The listing builds one solid part. Answer for the finished solid, in the listing's coordinates (mm). A direction names the side the tool comes from. Give positions to 0.01 mm unless a question says otherwise; leave off trailing zeros. Write each loop counter-clockwise with the first axis right and the second up, starting at its lowest first coordinate (ties: lowest second). Pieces come first, ordered by that corner, then holes. Notation, with made-up numbers: (62.5, -28.5) -> (83.5, -28.5) arc R24 cw to (83.5, -15.5) -> close; hole circle Ø1 at (-38.75, 55). An arc over 180 degrees is marked (long way). Use CSV: the item, a comma, the result in double quotes. Start each with the question number.
from build123d import *

# Parameters (mm, degrees)
SKETCH1_R           = 5.08
BOSS_EXTRUDE1_DEPTH = 7.62
SKETCH2_W           = 15.638324702
SKETCH2_H           = 10.16
CUT_EXTRUDE1_DEPTH  = 87.890649094
FILLET1_R           = 12.7
FILLET2_R           = 5.08


with BuildPart() as part:
    # Sketch1 → Boss-Extrude1 (new, symmetric)
    with BuildSketch(Plane(origin=(0, 0, 0), x_dir=(1, 0, 0), z_dir=(0, 1, 0))):
        with BuildLine():
            Line((2.735663722, 7.112), (8.018324702, 5.08))
            Line((8.018324702, 5.08), (8.018324702, 3.81))
            Line((8.018324702, 3.81), (68.181675298, 3.81))
            Line((68.181675298, 3.81), (68.181675298, 5.08))
            Line((68.181675298, 5.08), (73.464336278, 7.112))
            ThreePointArc((73.464336278, 7.112), (83.82, 0), (73.464336278, -7.112))
            Line((73.464336278, -7.112), (68.181675298, -5.08))
            Line((68.181675298, -5.08), (68.181675298, -3.81))
            Line((68.181675298, -3.81), (8.018324702, -3.81))
            Line((8.018324702, -3.81), (8.018324702, -5.08))
            Line((8.018324702, -5.08), (2.735663722, -7.112))
            ThreePointArc((2.735663722, -7.112), (-7.62, 0), (2.735663722, 7.112))
        make_face()
        with Locations(Location((0, 0, 0), (0, 0, 90))):
            Circle(SKETCH1_R, mode=Mode.SUBTRACT)
        with Locations(Location((76.2, 0, 0), (0, 0, 90))):
            Circle(SKETCH1_R, mode=Mode.SUBTRACT)
    extrude(amount=BOSS_EXTRUDE1_DEPTH, both=True)

    # Sketch2 → Cut-Extrude1 (cut, through all)
    with BuildSketch(Plane.XY.offset(13.97)):
        Polygon((8.018324702, 7.62), (68.181675298, 0), (83.82, 0), (83.82, 7.62), align=None)
        with Locations((0.199162351, 0)):
            Rectangle(SKETCH2_W, SKETCH2_H)
    extrude(amount=-CUT_EXTRUDE1_DEPTH, mode=Mode.SUBTRACT)

    # Fillet1
    # the kernel refuses this fillet: 12.7 mm, written as the material it adds along each edge
    with BuildSketch(Plane(origin=(68.181675298, 13.839504146, 3.81), x_dir=(-1, 0, 0), z_dir=(0, -1, 0))) as fillet1_piece_1_section:
        with BuildLine():
            CenterArc((5.535801658, -12.7), FILLET1_R, 90, 25.841932763)
            Line((0, -1.27), (0, 0))
            Line((0, 0), (5.535801658, 0))
        make_face()
    fillet1_piece_1 = extrude(amount=21.459504146, mode=Mode.PRIVATE)
    fillet1_piece_1 = split(fillet1_piece_1, bisect_by=Plane(origin=(64.458294063, 0.471585521, 3.912132652), z_dir=(-0.12565136927087708, -0.9920744596048997, 0)), keep=Keep.TOP, mode=Mode.PRIVATE)
    add(fillet1_piece_1)
    with BuildSketch(Plane(origin=(68.181675298, 13.839504146, -3.81), x_dir=(0, 0, -1), z_dir=(0, -1, 0))) as fillet1_piece_2_section:
        with BuildLine():
            CenterArc((12.7, -5.535801658), FILLET1_R, 154.158067237, 25.841932763)
            Line((0, -5.535801658), (0, 0))
            Line((0, 0), (1.27, 0))
        make_face()
    fillet1_piece_2 = extrude(amount=21.459504146, mode=Mode.PRIVATE)
    fillet1_piece_2 = split(fillet1_piece_2, bisect_by=Plane(origin=(67.224480553, 0.121233673, -4.63296), z_dir=(-0.12565136927087708, -0.9920744596048997, 0)), keep=Keep.TOP, mode=Mode.PRIVATE)
    add(fillet1_piece_2)
    with BuildSketch(Plane(origin=(8.018324702, 8.759504146, -3.81), x_dir=(1, 0, 0), z_dir=(0, -1, 0))) as fillet1_piece_3_section:
        with BuildLine():
            CenterArc((5.535801658, -12.7), FILLET1_R, 90, 25.841932763)
            Line((0, -1.27), (0, 0))
            Line((0, 0), (5.535801658, 0))
        make_face()
    fillet1_piece_3 = extrude(amount=30.219008291, mode=Mode.PRIVATE)
    fillet1_piece_3 = split(fillet1_piece_3, bisect_by=Plane(origin=(11.757033309, 5.08, -3.912132652), z_dir=(0, 1, 0)), keep=Keep.TOP, mode=Mode.PRIVATE)
    fillet1_piece_3 = split(fillet1_piece_3, bisect_by=Plane(origin=(11.871985872, 7.131913851, -3.912132652), z_dir=(-0.12565136927087708, -0.9920744596048997, 0)), keep=Keep.TOP, mode=Mode.PRIVATE)
    add(fillet1_piece_3)
    with BuildSketch(Plane(origin=(8.018324702, -5.08, -3.81), x_dir=(1, 0, 0), z_dir=(0, -1, 0))) as fillet1_piece_4:
        with BuildLine():
            CenterArc((5.535801658, -12.7), FILLET1_R, 90, 25.841932763)
            Line((0, -1.27), (0, 0))
            Line((0, 0), (5.535801658, 0))
        make_face()
    extrude(amount=2.54)
    with BuildSketch(Plane(origin=(8.018324702, 21.459504146, -3.81), x_dir=(0, 0, -1), z_dir=(0, -1, 0))) as fillet1_piece_5_section:
        with BuildLine():
            CenterArc((12.7, 5.535801658), FILLET1_R, 180, 25.841932763)
            Line((0, 5.535801658), (0, 0))
            Line((0, 0), (1.27, 0))
        make_face()
    fillet1_piece_5 = extrude(amount=16.379504146, mode=Mode.PRIVATE)
    fillet1_piece_5 = split(fillet1_piece_5, bisect_by=Plane(origin=(9.128609354, 7.479376698, -4.63296), z_dir=(-0.12565136927087708, -0.9920744596048997, 0)), keep=Keep.TOP, mode=Mode.PRIVATE)
    add(fillet1_piece_5)
    with BuildSketch(Plane(origin=(8.018324702, 21.459504146, -3.81), x_dir=(0, 0, -1), z_dir=(0, -1, 0))) as fillet1_piece_6_section:
        with BuildLine():
            CenterArc((12.7, 5.535801658), FILLET1_R, 180, 25.841932763)
            Line((0, 5.535801658), (0, 0))
            Line((0, 0), (1.27, 0))
        make_face()
    fillet1_piece_6 = extrude(amount=30.219008291, mode=Mode.PRIVATE)
    fillet1_piece_6 = split(fillet1_piece_6, bisect_by=Plane(origin=(8.985567945, -7.62, -4.63296), z_dir=(0, 1, 0)), keep=Keep.TOP, mode=Mode.PRIVATE)
    fillet1_piece_6 = split(fillet1_piece_6, bisect_by=Plane(origin=(8.985567945, -5.08, -4.63296), z_dir=(0, -1, 0)), keep=Keep.TOP, mode=Mode.PRIVATE)
    add(fillet1_piece_6)
    with BuildSketch(Plane(origin=(8.018324702, 21.459504146, 3.81), x_dir=(0, 0, 1), z_dir=(0, -1, 0))) as fillet1_piece_7_section:
        with BuildLine():
            CenterArc((12.7, -5.535801658), FILLET1_R, 154.158067237, 25.841932763)
            Line((0, -5.535801658), (0, 0))
            Line((0, 0), (1.27, 0))
        make_face()
    fillet1_piece_7 = extrude(amount=16.379504146, mode=Mode.PRIVATE)
    fillet1_piece_7 = split(fillet1_piece_7, bisect_by=Plane(origin=(9.128609354, 7.479376698, 4.63296), z_dir=(-0.12565136927087708, -0.9920744596048997, 0)), keep=Keep.TOP, mode=Mode.PRIVATE)
    add(fillet1_piece_7)
    with BuildSketch(Plane(origin=(8.018324702, 21.459504146, 3.81), x_dir=(0, 0, 1), z_dir=(0, -1, 0))) as fillet1_piece_8_section:
        with BuildLine():
            CenterArc((12.7, -5.535801658), FILLET1_R, 154.158067237, 25.841932763)
            Line((0, -5.535801658), (0, 0))
            Line((0, 0), (1.27, 0))
        make_face()
    fillet1_piece_8 = extrude(amount=30.219008291, mode=Mode.PRIVATE)
    fillet1_piece_8 = split(fillet1_piece_8, bisect_by=Plane(origin=(8.985567945, -7.62, 4.63296), z_dir=(0, 1, 0)), keep=Keep.TOP, mode=Mode.PRIVATE)
    fillet1_piece_8 = split(fillet1_piece_8, bisect_by=Plane(origin=(8.985567945, -5.08, 4.63296), z_dir=(0, -1, 0)), keep=Keep.TOP, mode=Mode.PRIVATE)
    add(fillet1_piece_8)
    with BuildSketch(Plane(origin=(8.018324702, 8.759504146, 3.81), x_dir=(0, 0, 1), z_dir=(0, -1, 0))) as fillet1_piece_9_section:
        with BuildLine():
            CenterArc((12.7, -5.535801658), FILLET1_R, 154.158067237, 25.841932763)
            Line((0, -5.535801658), (0, 0))
            Line((0, 0), (1.27, 0))
        make_face()
    fillet1_piece_9 = extrude(amount=30.219008291, mode=Mode.PRIVATE)
    fillet1_piece_9 = split(fillet1_piece_9, bisect_by=Plane(origin=(8.985567945, 5.08, 4.63296), z_dir=(0, 1, 0)), keep=Keep.TOP, mode=Mode.PRIVATE)
    fillet1_piece_9 = split(fillet1_piece_9, bisect_by=Plane(origin=(9.128609354, 7.479376698, 4.63296), z_dir=(-0.12565136927087708, -0.9920744596048997, 0)), keep=Keep.TOP, mode=Mode.PRIVATE)
    add(fillet1_piece_9)
    with BuildSketch(Plane(origin=(8.018324702, -5.08, 3.81), x_dir=(0, 0, 1), z_dir=(0, -1, 0))) as fillet1_piece_10:
        with BuildLine():
            CenterArc((12.7, -5.535801658), FILLET1_R, 154.158067237, 25.841932763)
            Line((0, -5.535801658), (0, 0))
            Line((0, 0), (1.27, 0))
        make_face()
    extrude(amount=2.54)

    # Fillet2
    # the kernel refuses this fillet: 5.08 mm, written as the material it takes off along each edge
    with BuildSketch(Plane(origin=(8.018324702, 5.08, -3.81), x_dir=(0, 0, 1), z_dir=(0, -1, 0)), Plane(origin=(8.018324702, 5.08, 3.81), x_dir=(1, 0, 0), z_dir=(0, -1, 0))) as fillet2_piece_1:
        with BuildLine():
            CenterArc((FILLET2_R, -FILLET2_R), FILLET2_R, 90, 90)
            Line((0, -FILLET2_R), (0, 0))
            Line((0, 0), (FILLET2_R, 0))
        make_face()
    extrude(amount=10.16, mode=Mode.SUBTRACT)


solid = part.part
Q1. Section C-C on y = -3 is taken. Give the vertices of the cut face in (x, z), then the cut area to 3 significant figures.
Q2. For faces 5 (the face through (-7.617, 6.368, 0.207)), 6 (the face through (5.34, -6.33, -6.11)), 7 (the face through (70.86, -3.76, 6.11)), determine the directions among +Z, -Z, +X, -X, +Y, -Y from which every point of the face is accessible in a straight line to the end or side of a thin tool.
Q3. Straight lines are drawn through the part: L1, parallel to X at y = -5.25, z = -1.25; L2, parallel to Z at x = 76.2, y = -3. For each, find the intervals that lie inside material, in ascending order.
Q4. The mould has two halves that part along Y. Classify faces 1 (the face through (9.951, 0.071, -2.717)), 2 (the face through (5, 5.08, 2)), 3 (the face through (70.7, 0, 0.1)), 4 (the face through (-5.037, -6.368, 0.661)): +Y half, -Y half, draft (parallel to the pull), parting line (faces both ways), or undercut.
Q5. Section B-B on x = 76.2 is taken. Give the vertices of the cut face in (y, z), then the cut area to 3 significant figures.
Q6. Flat-ended cylindrical pins translate along their axes: pin 1 Ø1 at (y, z) = (1, 4.5) entering from -X; pin 2 Ø5 at (x, z) = (72.5, 0.5) entering from -Y; pin 3 Ø8 at (y, z) = (0, 4.5) entering from -X; pin 4 Ø1 at (x, y) = (30, 1.5) entering from -Z. Find the tip coordinate at first contact, or state that the pin passes through.
Q7. Section A-A on x = 0 is taken. Give the vertices of the cut face in (y, z).
Q8. Section D-D on z = -2.5 is taken. Give the vertices of the cut face in (x, y), then the cut area to 3 significant figures.
Output:
1,outline,"(8.18, 0) arc R5.08 ccw to (13.1, -3.81) -> (62.65, -3.81) arc R12.7 cw to (68.18, -5.08) -> (73.46, -7.11) arc R7.62 ccw (long way) to (73.46, 7.11) -> (68.18, 5.08) arc R12.7 cw to (62.65, 3.81) -> (13.1, 3.81) arc R5.08 ccw to start; hole circle Ø10.16 at (76.2, 0)"
1,area,"567 mm²"
2,face 5,"+Y, -Y"
2,face 6,"-Z, +Y, -Y"
2,face 7,"+Z, +Y, -Y"
3,L1,"-7.52 to -4.92, 4.92 to 71.28, 81.12 to 83.72"
3,L2,"-7.62 to -5.08, 5.08 to 7.62"
4,face 1,"undercut"
4,face 2,"undercut"
4,face 3,"+Y half"
4,face 4,"draft"
5,outline,"(-7.62, -7.62) -> (0, -7.62) -> (0, -5.08) -> (-7.62, -5.08) -> close; (-7.62, 5.08) -> (0, 5.08) -> (0, 7.62) -> (-7.62, 7.62) -> close"
5,area,"38.7 mm²"
6,pin 1,"through"
6,pin 2,"y = -7.62"
6,pin 3,"x = 8.34"
6,pin 4,"z = -3.81"
7,outline,"(-7.62, -7.62) -> (-5.08, -7.62) -> (-5.08, -5.08) -> (-7.62, -5.08) -> close; (-7.62, 5.08) -> (-5.08, 5.08) -> (-5.08, 7.62) -> (-7.62, 7.62) -> close; (5.08, -7.62) -> (7.62, -7.62) -> (7.62, -5.08) -> (5.08, -5.08) -> close; (5.08, 5.08) -> (7.62, 5.08) -> (7.62, 7.62) -> (5.08, 7.62) -> close"
8,outline,"(-7.2, -7.62) -> (-4.42, -7.62) -> (-4.42, -5.08) -> (-7.2, -5.08) -> close; (-7.2, 5.08) -> (-4.42, 5.08) -> (-4.42, 7.62) -> (-7.2, 7.62) -> close; (4.42, -7.62) -> (71.78, -7.62) -> (71.78, 0) -> (68.18, 0) -> (8.02, 7.62) -> (4.42, 7.62) -> (4.42, 5.08) -> (9.69, 5.08) -> (9.69, -5.08) -> (4.42, -5.08) -> close; (80.62, -7.62) -> (83.4, -7.62) -> (83.4, 0) -> (80.62, 0) -> close"
8,area,"752 mm²"
